Study the drawing (mm; zero at the part's minimum x, y, z) and answer. Give positions to 0.01 mm unless a question says otherwise; leave off trailing zeros. Write each loop counter-clockwise with the first axis right and the second up, starting at its lowest first coordinate (ties: lowest second). Pieces come first, ordered by that corner, then holes. Notation, with made-up numbers: (63, 6.25) - (82, 6.25) arc R25 ccw to (82, 42.25) - close; hole circle Ø5 at (38, 6.25). An arc over 180 degrees is marked (long way). Return JSON: item names as keys, results as strings.
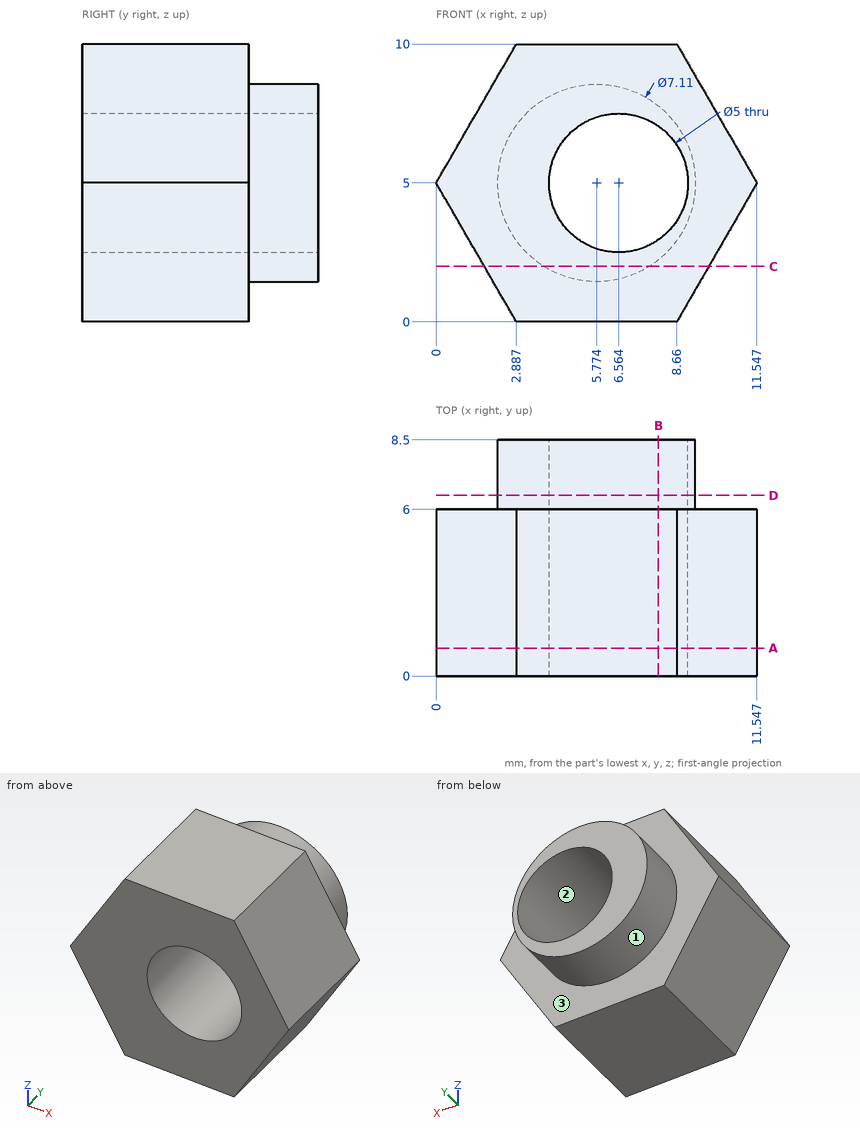
Item 1: A cutting plane is placed at B-B on x = 8. Determine the outline of the cut face in (y, z).
Answer below:
{"outline": "(0, 0) - (6, 0) - (6, 2.23) - (8.5, 2.23) - (8.5, 2.95) - (0, 2.95) - close; (0, 7.05) - (8.5, 7.05) - (8.5, 7.77) - (6, 7.77) - (6, 10) - (0, 10) - close"}
Item 2: A cutting plane is placed at C-C on z = 2. Determine the outline of the cut face in (x, y) (1 decimal).
Answer below:
{"outline": "(1.7, 0) - (9.8, 0) - (9.8, 6) - (7.7, 6) - (7.7, 8.5) - (3.9, 8.5) - (3.9, 6) - (1.7, 6) - close"}
Item 3: Flat-ended cylindrical pins translate along their axes: P1, Ø2, axis at y = 6.5, z = 2.5, coming from the -X side; P2, Ø1.5, axis at y = 3.5, z = 2, coming from the -X side. Find the tip coordinate at first contact, or state that the pin passes through.
Answer below:
{"P1": "stops at x = 0.94", "P2": "stops at x = 1.3"}
Item 4: The mould has two halves that part along X. Classify the marked faces 1, 2 and 3: +X half, -X half, draft (parallel to the pull), parting line (faces both ways), or undercut.
Answer below:
{"face 1": "parting line", "face 2": "undercut", "face 3": "draft"}
Item 5: A cutting plane is placed at D-D on y = 6.5. Determine the outline of the cut face in (x, z) (1 decimal).
Answer below:
{"outline": "circle Ø7.1 at (5.8, 5); hole circle Ø5 at (6.6, 5)"}
Item 6: A cutting plane is placed at A-A on y = 1. Determine the outline of the cut face in (x, z).
Answer below:
{"outline": "(0, 5) - (2.89, 0) - (8.66, 0) - (11.55, 5) - (8.66, 10) - (2.89, 10) - close; hole circle Ø5 at (6.56, 5)"}
Item 7: Consider L1, parallel to X at y = 7, z = 5; L2, parallel to Y at x = 3.25, z = 9; L3, parallel to Z at x = 8.5, y = 4.75. Determine where each line is inside the solid, lowest interval first.
Answer below:
{"L1": "x = 2.22 to 4.06, 9.06 to 9.33", "L2": "y = 0 to 6", "L3": "z = 0 to 3.42, 6.58 to 10"}
